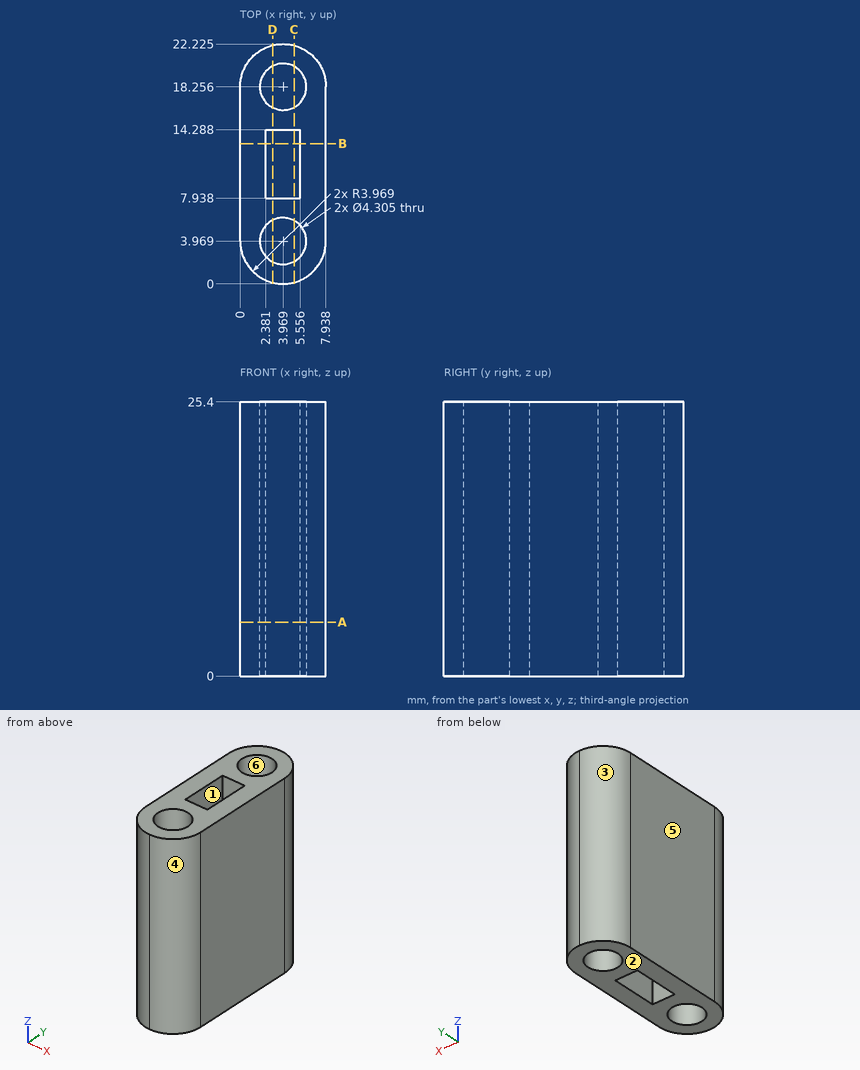
Input: dimensioned drawing with shaded views. Units: mm. Origin: part minimum x, y, z. A direction names the side the tool comes from. Give positions to 0.01 mm unless a question says otherwise; leave off trailing zeros. Write each loop counter-clockwise with the first axis right and the second up, starting at its lowest first coordinate (ties: lowest second). Pieces come first, ordered by that corner, then holes.
Q1. Section D-D, the plane x = 3. Output: boundary loops of the cut face in (y, z) (1 decimal), plus the area to 3 significant figures.
Q2. Section A-A, the plane z = 5. State how many separate pieces and enclosed holes the cut face has, plus the area to 3 significant figures.
Q3. Section B-B, the plane y = 13. Output: boundary loops of the cut face in (x, z), plus the area to 3 significant figures.
Q4. Pull-direction query (Y, two-part tool) for the marked faces 3, 4, 5 and 6; classes: pulls with the +Y half, pulls with the -Y half, needs draft (parallel to the pull), parting line crosses it, or undercut.
Q5. First-contact query: P1, Ø2, axis at x = 1, z = 21, coming from the +Y side; P2, Ø3, axis at x = 1, z = 4, coming from the -Y side. Flat tips, straight axial feed; report the tip coordinate or a pass-through.
Q6. Section C-C, the plane x = 5. Output: boundary loops of the cut face in (y, z) (1 decimal).
Q7. Set-up query: the marked faces 1 and 2. Return all of +Z, -Z, +X, -X, +Y, -Y with unobstructed straight access to the full face (end or side cutting, diameter ignored); none if empty.
Q8. Material intervals for probe 1 along X at (y, z) = (11.25, 3.5); probe 2 along Y at (x, z) = (4, 5.5) (1 decimal); probe 3 along Y at (x, z) = (2, 11) (1 decimal), sorted ascending.
Filled in:
1. outline: (0.1, 0) - (2, 0) - (2, 25.4) - (0.1, 25.4) - close; (5.9, 0) - (7.9, 0) - (7.9, 25.4) - (5.9, 25.4) - close; (14.3, 0) - (16.3, 0) - (16.3, 25.4) - (14.3, 25.4) - close; (20.2, 0) - (22.1, 0) - (22.1, 25.4) - (20.2, 25.4) - close
1. area: 202 mm2
2. separate pieces: 1
2. enclosed holes: 3
2. area: 114 mm2
3. outline: (0, 0) - (2.38, 0) - (2.38, 25.4) - (0, 25.4) - close; (5.56, 0) - (7.94, 0) - (7.94, 25.4) - (5.56, 25.4) - close
3. area: 121 mm2
4. face 3: pulls with the +Y half
4. face 4: pulls with the -Y half
4. face 5: needs draft
4. face 6: undercut
5. P1: stops at y = 21.7
5. P2: stops at y = 0.28
6. outline: (0.1, 0) - (2.1, 0) - (2.1, 25.4) - (0.1, 25.4) - close; (5.9, 0) - (7.9, 0) - (7.9, 25.4) - (5.9, 25.4) - close; (14.3, 0) - (16.4, 0) - (16.4, 25.4) - (14.3, 25.4) - close; (20.1, 0) - (22.1, 0) - (22.1, 25.4) - (20.1, 25.4) - close
7. face 1: +Z, -Z
7. face 2: -Z, +X, -X, +Y, -Y
8. probe 1: x = 0 to 2.38, 5.56 to 7.94
8. probe 2: y = 0 to 1.8, 6.1 to 7.9, 14.3 to 16.1, 20.4 to 22.2
8. probe 3: y = 0.5 to 3.1, 4.8 to 17.4, 19.1 to 21.7
